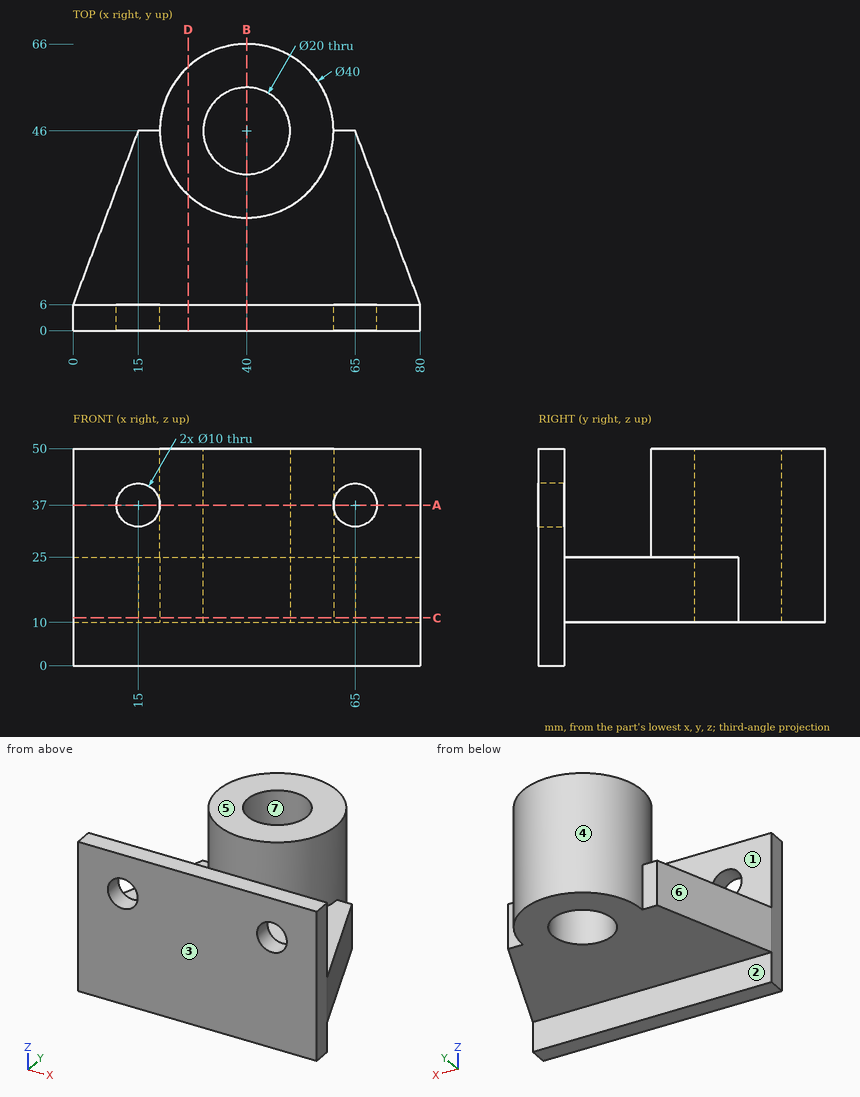
For this review, use the dimensioned drawing (mm, ordinates from the lowest corner) and the shaded views. A direction names the side the tool comes from. Coordinates: 2 decimals unless noted, no trailing zeros. Write each loop counter-clockwise with the first axis right and the second up, starting at its lowest first coordinate (ties: lowest second). Pieces come first, ordered by that corner, then holes. Notation, with made-up numbers: (66, 35.5) - (106, 35.5) arc R20 ccw to (106, 48.5) - close; hole circle Ø4 at (-0.5, 22). An arc over 180 degrees is marked (long way). Answer as a JSON object with one key per item and string values. Group by question number.
1. Mouldability with a two-part tool opening along X and no side actions: class the marked faces 5, 6 and 7 as pulls with the +X half, pulls with the -X half, needs draft (parallel to the pull), parting line crosses it, or undercut.
2. Add section C-C (z = 11). Give the boundary of the cut face in (x, y).
3. Clearance check with flat-ended pins moving along their axes: pin 1 Ø5 at (x, y) = (56.5, 32.5) entering from -Z; pin 2 Ø20 at (x, z) = (50, 37) entering from +Y; pin 3 Ø5.5 at (x, z) = (16.5, 20.5) entering from +Y. State where each tip first meets the part, or that it passes through.
4. Add section B-B (x = 40). Give the boundary of the cut face in (y, z).
5. To check wall thickness, follow probe 1 along X at (y, z) = (2.55, 37); probe 2 along Y at (x, z) = (34, 35); probe 3 along Z at (x, y) = (18.5, 43). State the ranges of each line that lie inside material, in increasing order.
6. Add section D-D (x = 26.5). Give the boundary of the cut face in (y, z).
7. Add section A-A (z = 37). Give the boundary of the cut face in (x, y), plus the area to 3 significant figures.
8. Machinability: for the marked faces 1, 2, 3 and 4, which of the approach directions +Z, -Z, +X, -X, +Y, -Y give a long, thin tool a straight path to every point of the face, cutting with its end or side? Answer none if there is none.
Findings:
{
 "1": {"face 5": "needs draft", "face 6": "pulls with the -X half", "face 7": "undercut"},
 "2": {"outline": "(0, 0) - (80, 0) - (80, 6) - (65, 46) - (60, 46) arc R20 ccw to (20, 46) - (15, 46) - (0, 6) - close; hole circle Ø20 at (40, 46)"},
 "3": {"pin 1": "z = 10", "pin 2": "y = 66", "pin 3": "y = 46"},
 "4": {"outline": "(0, 0) - (6, 0) - (6, 10) - (36, 10) - (36, 50) - (26, 50) - (26, 25) - (6, 25) - (6, 50) - (0, 50) - close; (56, 10) - (66, 10) - (66, 50) - (56, 50) - close"},
 "5": {"probe 1": "0 to 10, 20 to 60, 70 to 80", "probe 2": "0 to 6, 26.92 to 38, 54 to 65.08", "probe 3": "10 to 25"},
 "6": {"outline": "(0, 0) - (6, 0) - (6, 10) - (60.76, 10) - (60.76, 50) - (31.24, 50) - (31.24, 25) - (6, 25) - (6, 50) - (0, 50) - close"},
 "7": {"outline": "(0, 0) - (10, 0) - (10, 6) - (0, 6) - close; (20, 0) - (60, 0) - (60, 6) - (20, 6) - close; circle Ø40 at (40, 46); (70, 0) - (80, 0) - (80, 6) - (70, 6) - close; hole circle Ø20 at (40, 46)", "area": "1,300 mm²"},
 "8": {"face 1": "+Z, +X, -X", "face 2": "-Z, +X, -X, +Y", "face 3": "+Z, -Z, +X, -X, -Y", "face 4": "+Z"}
}
